Work out the finished part from the listing and answer in its coordinate system (mm). A direction names the side the tool comes from. Coordinates: 2 decimals unless noted, no trailing zeros. Write each loop counter-clockwise with the first axis right and the second up, starting at its lowest first coordinate (ties: lowest second). Pieces come first, ordered by that corner, then holes. Notation, with made-up numbers: (87, 77) - (134, 77) arc R24 ccw to (134, 87) - close; hole circle Ø4 at (41.25, 82). An arc over 180 degrees is marked (long way). Use a Markdown table: item, result. Add a question column.
(1) The part is cut by section A-A, the plane y = 63. Give the vertices of the cut face in (x, z), then the cut area to 3 significant figures.
(2) The part is cut by section C-C, the plane z = 12.5. Give the vertices of the cut face in (x, y).
(3) Find the intervals of material crossed by line 1 (Y direction, x = 37.5, z = 52.5); line 2 (Y direction, x = 21, z = 47); line 3 (X direction, y = 63, z = 32), in increasing order. Write a range as from..to.
(4) Given pin 1 Ø1.5 at (x, y) = (54.5, 10.5) entering from +Z; pin 2 Ø6 at (x, y) = (62.5, 58) entering from +Z; pin 3 Ø7.5 at (x, z) = (18, 47.5) entering from -Y; pin 4 Ø5 at (y, z) = (18.5, 11.5) entering from -X, each flat-ended and moving along its own axis, determine where each tip first touches the part or whether it passes through.
(5) A tool of negligible diameter and unlimited length cuts with its end or side. For faces 1 (the face through (37, 51, 58)), 2 (the face through (13, 40, 47)), 3 (the face through (27, 0, 8)), 4 (the face through (50, 60, 38)), from which of +Z, -Z, +X, -X, +Y, -Y can it reach the whole face along a straight path? Write none if from no direction.
(6) The part is cut by section B-B, the plane x = 19.5. Give the vertices of the cut face in (y, z), then the cut area to 3 significant figures.
(7) The part is cut by section D-D, the plane y = 8. Give the vertices of the cut face in (x, z), then the cut area to 3 significant figures.
from build123d import *

# Parameters (mm, degrees)
F0_W          = 70
F0_H          = 70
F1_DEPTH      = 60
F3_DEPTH      = 70.001
F4_W          = 50
F4_H          = 50
F5_DEPTH      = 40
F6_SIZE       = 10
F7_W          = 20
F7_H          = 40
F8_DEPTH      = 20
F9_R          = 5
F10_T1_DEPTH  = 32.5
F10_T3_DEPTH  = 15
F10_S7_W      = 5
F10_S7_H      = 5
F10_T8_DEPTH  = 5
F10_T12_ANGLE = 90


# Not quite as in the source:
# - a fillet or chamfer that OpenCascade refuses, or shapes differently, is made with other operations: its cross-section is extruded or revolved along the edge and cut away or added


with BuildPart() as f1:
    # F0 (on Top) → F1 (new body)
    with BuildSketch(Plane.XY):
        with Locations((35, 35)):
            Rectangle(F0_W, F0_H)
    extrude(amount=F1_DEPTH)

    # F2 (on face) → F3 (cut, through all)
    with BuildSketch(Plane.YZ.offset(70)):
        with BuildLine():
            Line((40, 60), (0, 60))
            Line((0, 60), (0, 20))
            Line((0, 20), (20, 20))
            ThreePointArc((20, 20), (34.1421356237, 25.8578643763), (40, 40))
            Line((40, 40), (40, 60))
        make_face()
    extrude(amount=-F3_DEPTH, mode=Mode.SUBTRACT)

    # F4 (on face) → F5 (cut)
    with BuildSketch(Plane.YZ.offset(70)):
        with Locations((25, 35)):
            Rectangle(F4_W, F4_H)
    extrude(amount=-F5_DEPTH, mode=Mode.SUBTRACT)

    # F6
    f6_edges = [f1.edges().sort_by_distance(p)[0] for p in [
        (50, 50, 10),
    ]]
    chamfer(f6_edges, length=F6_SIZE)

    # F7 (on face) → F8 (cut)
    with BuildSketch(Plane.YZ.offset(70)):
        with Locations((60, 40)):
            Rectangle(F7_W, F7_H)
    extrude(amount=-F8_DEPTH, mode=Mode.SUBTRACT)

    # F9
    f9_edges = [f1.edges().sort_by_distance(p)[0] for p in [
        (40, 50, 60),
        (30, 45, 60),
        (15, 40, 60),
        (0, 55, 60),
        (25, 70, 60),
        (50, 60, 60),
    ]]
    fillet(f9_edges, radius=F9_R)

    # F10: fillet of radius 5 on 1 edges, made by hand

    # F10_s2 → F10_t1 (cut)
    with BuildSketch(Plane.XZ.offset(-20)):
        with BuildLine():
            ThreePointArc((25, 20), (28.5355339059, 18.5355339059), (30, 15))
            Line((30, 15), (30, 20))
            Line((30, 20), (25, 20))
        make_face()
    extrude(amount=F10_T1_DEPTH, mode=Mode.SUBTRACT)

    # F10_s4 → F10_t3 (cut)
    with BuildSketch(Plane.XY.offset(40)):
        with BuildLine():
            ThreePointArc((25, 40), (28.5355339059, 41.4644660941), (30, 45))
            Line((30, 45), (30, 40))
            Line((30, 40), (25, 40))
        make_face()
    extrude(amount=F10_T3_DEPTH, mode=Mode.SUBTRACT)


with BuildPart() as f10_tool6:
    # F10_s7 → F10_t8 (new body)
    with BuildSketch(Plane.XZ.offset(-45)):
        with Locations((27.5, 57.5)):
            Rectangle(F10_S7_W, F10_S7_H)
    extrude(amount=F10_T8_DEPTH)

    # F10_s9 → F10_t10 (revolve, cut)
    with BuildSketch(Plane(origin=(25, 45, 55), x_dir=(-0.7071067812, 0, -0.7071067812), z_dir=(-0.7071067812, 0, 0.7071067812))):
        with BuildLine():
            ThreePointArc((0, -5), (5, 0), (0, 5))
            Line((0, 5), (0, -5))
        make_face()
    revolve(axis=Axis((25, 45, 55), (0, -1, 0)), mode=Mode.SUBTRACT)


with BuildPart() as f1_1:
    add(f1.part)

    # F10_t5: cut F10_tool6
    add(f10_tool6.part, mode=Mode.SUBTRACT)

    # F10_s11 → F10_t12 (revolve, cut)
    with BuildSketch(Plane.XZ.offset(-20)):
        with BuildLine():
            ThreePointArc((25, 20), (28.5355339059, 18.5355339059), (30, 15))
            Line((30, 15), (30, 20))
            Line((30, 20), (25, 20))
        make_face()
    revolve(axis=Axis((30, 20, 40), (1, 0, 0)), revolution_arc=F10_T12_ANGLE, mode=Mode.SUBTRACT)


solid = f1_1.part
Model answer:
| question | item | result |
|---|---|---|
| 1 | outline | (0, 0) - (70, 0) - (70, 20) - (50, 20) - (50, 55) arc R5 ccw to (45, 60) - (5, 60) arc R5 ccw to (0, 55) - close |
| 1 | area | 3,390 mm^2 |
| 2 | outline | (0, 0) - (30, 0) - (30, 42.5) - (70, 42.5) - (70, 70) - (0, 70) - close |
| 3 | line 1 | 50..70 |
| 3 | line 2 | 40..70 |
| 3 | line 3 | 0..50 |
| 4 | pin 1 | z = 10 |
| 4 | pin 2 | z = 20 |
| 4 | pin 3 | y = 40 |
| 4 | pin 4 | x = 0 |
| 5 | face 1 | +Z, +X, -Y |
| 5 | face 2 | +Z, +X, -X, -Y |
| 5 | face 3 | +Z, -Z, +X, -X, -Y |
| 5 | face 4 | +Z, +X, +Y, -Y |
| 6 | outline | (0, 0) - (70, 0) - (70, 55) arc R5 ccw to (65, 60) - (45, 60) arc R5 ccw to (40, 55) - (40, 40) arc R20 cw to (20, 20) - (0, 20) - close |
| 6 | area | 2,680 mm^2 |
| 7 | outline | (0, 0) - (70, 0) - (70, 10) - (30, 10) - (30, 15) arc R5 ccw to (25, 20) - (0, 20) - close |
| 7 | area | 995 mm^2 |
